The listing builds one solid part. Answer for the finished solid, in the listing's coordinates (mm). Face numbers are marked on the shaded views. A direction names the side the tool comes from. Give positions to 0.01 mm unless a question says otherwise; leave off trailing zeros. Write each loop counter-clockwise with the first axis right and the second up, starting at its lowest first coordinate (ties: lowest second). Pieces come first, ordered by that corner, then holes. Notation, with made-up numbers: (35, -23.5) - (45, -23.5) arc R13 ccw to (45, -4.5) - close; hole circle Ø3 at (46, 23.25). An arc over 180 degrees is marked (long way). Write each question's results on one line, items separated by ' | '. Start each with the question number.
Q1. Section C-C (y = 131.5) is taken. Determine the outline of the cut face in (x, z), plus the area to 3 significant figures.
Q2. For the marked faces 1 and 2, determine the directions among +Z, -Z, +X, -X, +Y, -Y from which every point of the face is accessible in a straight line to the end or side of a thin tool.
Q3. Find the intervals of material crossed by probe 1 along Y at (x, z) = (4.75, -6.25); probe 2 along X at (y, z) = (167, -0.75); probe 3 along X at (y, z) = (97, 6.75), in increasing order.
Q4. Section B-B (z = 2.75) is taken. Determine the outline of the cut face in (x, y).
Q5. Flat-ended cylindrical pins translate along their axes: pin 1 Ø2 at (y, z) = (98.5, 4) entering from -X; pin 2 Ø1.5 at (y, z) = (192, -3.5) entering from +X; pin 3 Ø3 at (y, z) = (182.5, 3) entering from +X. Find the tip coordinate at first contact, or state that the pin passes through.
Q6. Section A-A (x = 4.5) is taken. Determine the outline of the cut face in (y, z).
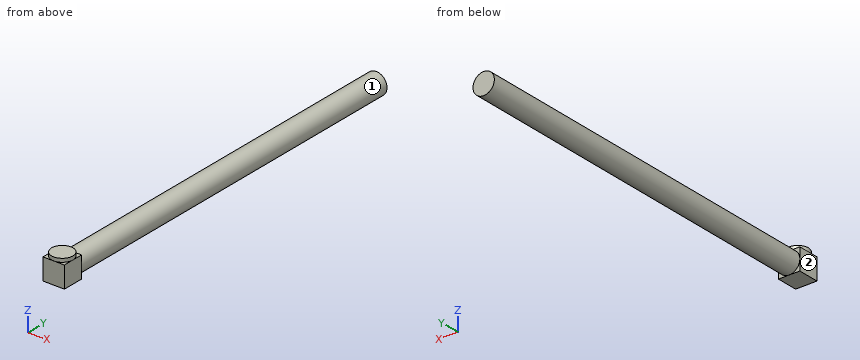
```python
from build123d import *

# Parameters (mm, degrees)
SKETCH1_R           = 7.5
BOSS_EXTRUDE1_DEPTH = 266.7
BOSS_EXTRUDE2_START = 15
SKETCH2_R           = 7.5
BOSS_EXTRUDE2_DEPTH = 15
SKETCH3_R           = 7.5
BOSS_EXTRUDE3_DEPTH = 2.5


with BuildPart() as part:
    # Sketch1 → Boss-Extrude1 (new body)
    with BuildSketch(Plane(origin=(0, 0, 0), x_dir=(1, 0, 0), z_dir=(0, 1, 0))):
        with Locations(Location((0, 0, 0), (0, 0, 270))):
            Circle(SKETCH1_R)
    extrude(amount=BOSS_EXTRUDE1_DEPTH)

    # Sketch2 → Boss-Extrude2 (add)
    with BuildSketch(Plane.XZ.offset(BOSS_EXTRUDE2_START)):
        with BuildLine():
            Line((0, 7.5), (-7.5, 7.5))
            Line((-7.5, 7.5), (-7.5, 0))
            ThreePointArc((-7.5, 0), (-5.303300859, 5.303300859), (0, 7.5))
        make_face()
        with Locations(Location((0, 0, 0), (0, 0, 90))):
            Circle(SKETCH2_R)
        with BuildLine():
            Line((7.5, 7.5), (0, 7.5))
            ThreePointArc((0, 7.5), (5.303300859, 5.303300859), (7.5, 0))
            Line((7.5, 0), (7.5, 7.5))
        make_face()
        with BuildLine():
            Line((7.5, -7.5), (7.5, 0))
            ThreePointArc((7.5, 0), (5.303300859, -5.303300859), (0, -7.5))
            Line((0, -7.5), (7.5, -7.5))
        make_face()
        with BuildLine():
            ThreePointArc((0, -7.5), (-5.303300859, -5.303300859), (-7.5, 0))
            Line((-7.5, 0), (-7.5, -7.5))
            Line((-7.5, -7.5), (0, -7.5))
        make_face()
    extrude(amount=-BOSS_EXTRUDE2_DEPTH)

    # Sketch3 → Boss-Extrude3 (add)
    with BuildSketch(Plane.XY.offset(7.5)):
        with Locations((0, -7.5)):
            Circle(SKETCH3_R)
    extrude(amount=BOSS_EXTRUDE3_DEPTH)


solid = part.part
```
Answers below:
1) outline: circle Ø15 at (0, 0) | area: 177 mm2
2) face 1: +Y | face 2: +Z, -Z, -X, +Y, -Y
3) probe 1: y = -15 to 0 | probe 2: x = -7.46 to 7.46 | probe 3: x = -3.27 to 3.27
4) outline: (-7.5, -15) - (7.5, -15) - (7.5, 0) - (6.98, 0) - (6.98, 266.7) - (-6.98, 266.7) - (-6.98, 0) - (-7.5, 0) - close
5) pin 1: stops at x = -6.87 | pin 2: stops at x = 6.98 | pin 3: stops at x = 7.35
6) outline: (-15, -7.5) - (0, -7.5) - (0, -6) - (266.7, -6) - (266.7, 6) - (0, 6) - (0, 7.5) - (-1.5, 7.5) - (-1.5, 10) - (-13.5, 10) - (-13.5, 7.5) - (-15, 7.5) - close
